Can you work these out from the model? Positions are in its coordinate system, mm. Face numbers are marked on the shaded views. A direction names the side the tool comes from. Round coordinates to 2 decimals unless told otherwise and drop trailing zeros. Loops run counter-clockwise (first coordinate to the right, second up) from the corner with the lowest first, then second, coordinate; pieces in that order, holes last. Notation, with made-up numbers: (-11.5, 32) - (18.5, 32) arc R11 ccw to (18.5, 44) - close; hole circle Ø2 at (88.25, 57). An arc over 180 degrees is marked (long way). Answer as CSV lines item,"result".
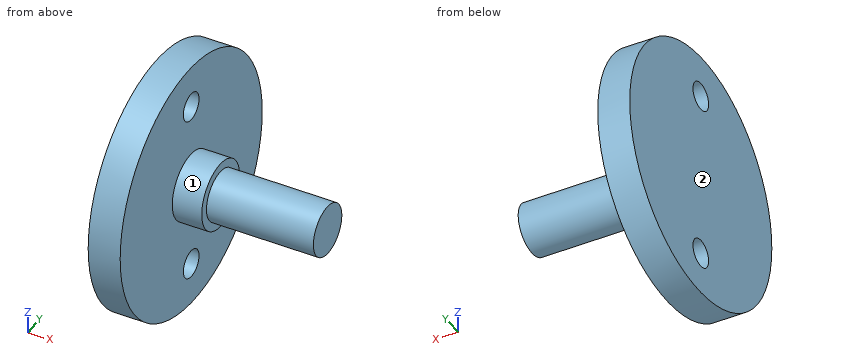
```python
from build123d import *

# Parameters (mm, degrees)
SKETCH_1_R          = 15
EXTRUDE_1_DEPTH     = 10.8
SKETCH_2_R          = 4
EXTRUDE_2_DEPTH     = 3.5
SKETCH_3_R          = 3
EXTRUDE_3_DEPTH     = 5.8
SKETCH_4_R          = 1.65
CUT_EXTRUDE_1_DEPTH = 30.223449488
SKETCH_5_R          = 3
EXTRUDE_4_DEPTH     = 6.9
SKETCH_6_R          = 15
CUT_EXTRUDE_2_DEPTH = 7


with BuildPart() as part:
    # ｽｹｯﾁ1 → ﾎﾞｽ - 押し出し1 (new body)
    with BuildSketch(Plane(origin=(0, 0, 0), x_dir=(0, 0, -1), z_dir=(1, 0, 0))):
        with Locations(Location((0, 0, 0), (0, 0, 180))):
            Circle(SKETCH_1_R)
    extrude(amount=EXTRUDE_1_DEPTH)

    # ｽｹｯﾁ2 → ﾎﾞｽ - 押し出し2 (add)
    with BuildSketch(Plane(origin=(10.8, 0, 0), x_dir=(0, 0, -1), z_dir=(1, 0, 0))):
        Circle(SKETCH_2_R)
    extrude(amount=EXTRUDE_2_DEPTH)

    # ｽｹｯﾁ3 → ﾎﾞｽ - 押し出し3 (add)
    with BuildSketch(Plane(origin=(14.3, 0, 0), x_dir=(0, 0, -1), z_dir=(1, 0, 0))):
        Circle(SKETCH_3_R)
    extrude(amount=EXTRUDE_3_DEPTH)

    # ｽｹｯﾁ4 → ｶｯﾄ - 押し出し1 (cut, through all)
    with BuildSketch(Plane.ZY):
        with Locations((10, 0)):
            Circle(SKETCH_4_R)
        with Locations(Location((-10, 0, 0), (0, 0, 180))):
            Circle(SKETCH_4_R)
    extrude(amount=-CUT_EXTRUDE_1_DEPTH, mode=Mode.SUBTRACT)

    # ｽｹｯﾁ5 → ﾎﾞｽ - 押し出し4 (add)
    with BuildSketch(Plane(origin=(20.1, 0, 0), x_dir=(0, 0, -1), z_dir=(1, 0, 0))):
        Circle(SKETCH_5_R)
    extrude(amount=EXTRUDE_4_DEPTH)

    # ｽｹｯﾁ6 → ｶｯﾄ - 押し出し2 (cut)
    with BuildSketch(Plane.ZY):
        Circle(SKETCH_6_R)
    extrude(amount=-CUT_EXTRUDE_2_DEPTH, mode=Mode.SUBTRACT)


solid = part.part
```
Q1. I'm going to push flat-ended pins straight in: pin 1 Ø1 at (x, y) = (11, 11.5) entering from -Z; pin 2 Ø3 at (y, z) = (-1, -6.5) entering from +X; pin 3 Ø5 at (x, y) = (9.5, 7.5) entering from -Z; pin 4 Ø2 at (y, z) = (0, 10) entering from +X. Where does each tip first touch, or does it pass through?
Checks:
pin 1,"z = -10.15"
pin 2,"x = 10.8"
pin 3,"z = -14.14"
pin 4,"through"
Q2. Imagine slicing it at D-D (y = -8.25). Write out the boundary of the cut face in (x, z), then the cut area to 3 significant figures.
Checks:
outline,"(7, -12.53) - (10.8, -12.53) - (10.8, 12.53) - (7, 12.53) - close"
area,"95.2 mm²"
Q3. Imagine slicing it at C-C (x = 22). Write out the boundary of the cut face in (y, z), then the cut area to 3 significant figures.
Checks:
outline,"circle Ø6 at (0, 0)"
area,"28.3 mm²"
Q4. Imagine slicing it at B-B (z = 10). Write out the boundary of the cut face in (x, y), then the cut area to 3 significant figures.
Checks:
outline,"(7, -11.18) - (10.8, -11.18) - (10.8, -1.65) - (7, -1.65) - close; (7, 1.65) - (10.8, 1.65) - (10.8, 11.18) - (7, 11.18) - close"
area,"72.4 mm²"
Q5. If I drill on line 1 along Y through (x, z) = (9.35, -10); line 2 along X through (y, z) = (-11.75, -5.25); line 3 along Z through (x, y) = (21.75, 1.25), over which ranges is the centre line in solid material (lowest first)? Write a range as [from, to].
Checks:
line 1,"[-11.18, -1.65], [1.65, 11.18]"
line 2,"[7, 10.8]"
line 3,"[-2.73, 2.73]"
Q6. Imagine slicing it at A-A (z = 0). Write out the boundary of the cut face in (x, y), then the cut area to 3 significant figures.
Checks:
outline,"(7, -15) - (10.8, -15) - (10.8, -4) - (14.3, -4) - (14.3, -3) - (27, -3) - (27, 3) - (14.3, 3) - (14.3, 4) - (10.8, 4) - (10.8, 15) - (7, 15) - close"
area,"218 mm²"
Q7. On a 3-axis mill with a long thin cutter (end or side, diameter ignored), from which of +Z, -Z, +X, -X, +Y, -Y can I reach the whole of each face in a straight line? I mean the marked faces 1 and 2. Say none if no direction works.
Checks:
face 1,"+X"
face 2,"+Z, -Z, -X, +Y, -Y"
